The listing builds one solid part. Answer for the finished solid, in the listing's coordinates (mm). A direction names the side the tool comes from. Coordinates: 2 decimals unless noted, no trailing zeros. Order: outer loops, then holes, each group sorted by start corner. A loop starts at its lowest first (then second) coordinate and runs counter-clockwise, first axis right, second up. Notation, with made-up numbers: (68.5, -20) -> (82.5, -20) arc R26 ccw to (82.5, 3) -> close; hole circle Ø11 at (-20, 77). An arc over 180 degrees is marked (long way). Return JSON: item names as keys, results as strings.
from build123d import *

# Parameters (mm, degrees)
SKETCH1_R           = 1.600000124
BOSS_EXTRUDE1_DEPTH = 9.8
SKETCH2_R           = 3.949999995
BOSS_EXTRUDE2_DEPTH = 1.2


with BuildPart() as part:
    # Sketch1 → Boss-Extrude1 (new body)
    with BuildSketch(Plane.XY.offset(11)):
        with BuildLine():
            Line((4.333958961, -10.506317019), (10.493660346, -4.364516586))
            ThreePointArc((10.493660346, -4.364516586), (14.560364187, -0.021186842), (10.506317019, 4.333958961))
            Line((10.506317019, 4.333958961), (4.364516586, 10.493660346))
            Line((4.364516586, 10.493660346), (-4.364516586, 10.493660346))
            Line((-4.364516586, 10.493660346), (-10.506317019, 4.333958961))
            ThreePointArc((-10.506317019, 4.333958961), (-14.560364187, -0.021186842), (-10.493660346, -4.364516586))
            Line((-10.493660346, -4.364516586), (-4.333958961, -10.506317019))
            Line((-4.333958961, -10.506317019), (4.333958961, -10.506317019))
        make_face()
        with Locations((11.217179708, -0.008876194)):
            Circle(SKETCH1_R, mode=Mode.SUBTRACT)
        with Locations((-11.217179708, -0.008876194)):
            Circle(SKETCH1_R, mode=Mode.SUBTRACT)
        Polygon((0, 8.900009778), (3.673546249, 8.905354887), (8.894626983, 3.699447494), (8.905354887, -3.673546249), (3.699447494, -8.894626983), (0, -8.900009778), (-3.699447494, -8.894626983), (-8.905354887, -3.673546249), (-8.894626983, 3.699447494), (-3.673546249, 8.905354887), align=None, mode=Mode.SUBTRACT)
    extrude(amount=-BOSS_EXTRUDE1_DEPTH)

    # Sketch2 → Boss-Extrude2 (add)
    with BuildSketch(Plane(origin=(0, 0, 1.2), x_dir=(-1, 0, 0), z_dir=(0, 0, -1))):
        with BuildLine():
            Line((4.364516586, 10.493660346), (-4.364516586, 10.493660346))
            Line((-4.364516586, 10.493660346), (-10.506317019, 4.333958961))
            ThreePointArc((-10.506317019, 4.333958961), (-14.560364187, -0.021186842), (-10.493660346, -4.364516586))
            Line((-10.493660346, -4.364516586), (-4.333958961, -10.506317019))
            Line((-4.333958961, -10.506317019), (4.333958961, -10.506317019))
            Line((4.333958961, -10.506317019), (10.493660346, -4.364516586))
            ThreePointArc((10.493660346, -4.364516586), (14.560364187, -0.021186842), (10.506317019, 4.333958961))
            Line((10.506317019, 4.333958961), (4.364516586, 10.493660346))
        make_face()
        Circle(SKETCH2_R, mode=Mode.SUBTRACT)
    extrude(amount=BOSS_EXTRUDE2_DEPTH)


solid = part.part
1. The part is cut by section D-D on x = -11.25. Give the vertices of the cut face in (y, z), and give its area (3 significant figures).
Answer block:
{"outline": "(-4.25, 0) -> (4.22, 0) -> (4.22, 11) -> (1.59, 11) -> (1.59, 1.2) -> (-1.61, 1.2) -> (-1.61, 11) -> (-4.25, 11) -> close", "area": "61.7 mm2"}
2. Determine the mould class of faces 1 (the face through (6.339, -6.248, 6.169)), 2 (the face through (-7, -6, 11)), 3 (the face through (-7.37, -7.48, 5.58)) for opening direction X: pulls with the +X half, pulls with the -X half, needs draft (parallel to the pull), parting line crosses it, or undercut.
Answer block:
{"face 1": "undercut", "face 2": "needs draft", "face 3": "pulls with the -X half"}
3. For faces 4 (the face through (0.856, -3.856, 0.608)), 5 (the face through (-6.266, -6.321, 6.169)), determine the directions among +Z, -Z, +X, -X, +Y, -Y from which every point of the face is accessible in a straight line to the end or side of a thin tool.
Answer block:
{"face 4": "+Z, -Z", "face 5": "+Z"}
4. The part is cut by section C-C on z = 7.5. Give the vertices of the cut face in (x, y), and give its area (3 significant figures).
Answer block:
{"outline": "(-10.51, 4.33) arc R4.36 ccw to (-10.49, -4.36) -> (-4.33, -10.51) -> (4.33, -10.51) -> (10.49, -4.36) arc R4.36 ccw to (10.51, 4.33) -> (4.36, 10.49) -> (-4.36, 10.49) -> close; hole circle Ø3.2 at (-11.22, -0.01); hole (-8.91, -3.67) -> (-3.7, -8.89) -> (0, -8.9) -> (3.7, -8.89) -> (8.91, -3.67) -> (8.89, 3.7) -> (3.67, 8.91) -> (0, 8.9) -> (-3.67, 8.91) -> (-8.89, 3.7) -> close; hole circle Ø3.2 at (11.22, -0.01)", "area": "141 mm2"}
5. Consider line 1 (Y direction, x = 0, z = 0.9); line 2 (Y direction, x = 2, z = 3.25); line 3 (X direction, y = 5.75, z = 8.5). Determine where each line is inside the solid, lowest interval first. Write a range as from..to.
Answer block:
{"line 1": "y = -10.51..-3.95, 3.95..10.49", "line 2": "y = -10.51..-8.9, 8.9..10.49", "line 3": "x = -9.09..-6.84, 6.84..9.09"}
6. The part is cut by section B-B on y = 2.75. Give the vertices of the cut face in (x, z).
Answer block:
{"outline": "(-13.57, 0) -> (-2.84, 0) -> (-2.84, 1.2) -> (-8.9, 1.2) -> (-8.9, 11) -> (-13.57, 11) -> close; (2.84, 0) -> (13.57, 0) -> (13.57, 11) -> (8.9, 11) -> (8.9, 1.2) -> (2.84, 1.2) -> close"}
7. Each of these flat-tipped pins is pushed along its axis until it touches: pin 1 Ø6 at (y, z) = (-6.5, 7) entering from -X; pin 2 Ø4 at (x, y) = (5, -2.5) entering from +Z. Where does it stop, or does it pass through?
Answer block:
{"pin 1": "stops at x = -12.82", "pin 2": "stops at z = 1.2"}
8. The part is cut by section A-A on x = -2. Give the vertices of the cut face in (y, z), and give its area (3 significant figures).
Answer block:
{"outline": "(-10.51, 0) -> (-3.41, 0) -> (-3.41, 1.2) -> (-8.9, 1.2) -> (-8.9, 11) -> (-10.51, 11) -> close; (3.41, 0) -> (10.49, 0) -> (10.49, 11) -> (8.9, 11) -> (8.9, 1.2) -> (3.41, 1.2) -> close", "area": "48.4 mm2"}
